Autodesk Fusion 360 part; units mm, degrees
sketch "Sketch1" plane through (0, 0, 0) normal (0, 0, 1) x (1, 0, 0)
  circle A0 centre (0, 0) radius 2.5
  dimension "d1" = 5
extrude "Extrude1" add sketch "Sketch1" along normal blind 20
sketch "Sketch2" plane through (0, 0, 20) normal (0, 0, 1) x (-1, 0, 0)
  circle A0 centre (0, 0) radius 2.5
  line L0 (-2.3094, 4) -> (-4.6188, 0)
  line L1 (-4.6188, 0) -> (-2.3094, -4)
  line L2 (-2.3094, -4) -> (2.3094, -4)
  line L3 (2.3094, -4) -> (4.6188, 0)
  line L4 (4.6188, 0) -> (2.3094, 4)
  line L5 (2.3094, 4) -> (-2.3094, 4)
  dimension "d4" = 4
extrude "Extrude2" add sketch "Sketch2" along normal blind 4 contours A0 | L0 L1 L2 L3 L4 L5
thread "Thread1"
Geometry: final body of the model. Coordinates: model frame, mm. A direction names the side the tool comes from. Round coordinates to 2 decimals unless told otherwise and drop trailing zeros. Loops run counter-clockwise (first coordinate to the right, second up) from the corner with the lowest first, then second, coordinate; pieces in that order, holes last. Notation, with made-up numbers: M 18.5,1.25 L 53.5,1.25 A12 ccw 53.5,24.25 Z; hole C 52.25,-27 d9. An arc over 180 degrees is marked long. One line per question, with ' | ' between items.
(1) Contact query for flat-ended pins moving along their axis: P1, Ø5, axis at x = 3, z = 11.5, coming from the +Y side; P2, Ø5, axis at x = -1.5, z = 13.5, coming from the -Y side; P3, Ø4, axis at x = -3, z = 8, coming from the +Y side. Output: stop coordinate, or through.
Check result:
P1: stops at y = 2.45 | P2: stops at y = -2.5 | P3: stops at y = 2.29
(2) Cut plane C-C on y = -1. Return the cut outline in (x, z), plus the area to 3 significant figures.
Check result:
outline: M -4.04,20 L -2.29,20 L -2.29,0 L 2.29,0 L 2.29,20 L 4.04,20 L 4.04,24 L -4.04,24 Z | area: 124 mm2
(3) Access query for faces 1 (the flat face through (-2, -2, 20)), 2 (the flat face through (0, 4, 22)). Directions: +Z, -Z, +X, -X, +Y, -Y. A direction counts if a zero-diameter tool reaches every point of the face in a straight line with its end or side. Return the directions, or none.
Check result:
face 1: -Z | face 2: +Z, -Z, +X, -X, +Y
(4) Material intervals for line 1 along Z through (x, y) = (2.25, 2.5); line 2 along Y through (x, z) = (1, 4.75); line 3 along X through (y, z) = (1.75, 9.5), sorted ascending. Write a range as from..to.
Check result:
line 1: z = 20..24 | line 2: y = -2.29..2.29 | line 3: x = -1.79..1.79
(5) Cut plane D-D on z = 3.25. Return the cut outline in (x, y).
Check result:
outline: C 0,0 d5
(6) Cut plane A-A on x = 0. Return the cut outline in (y, z), plus the area to 3 significant figures.
Check result:
outline: M -4,20 L -2.5,20 L -2.5,0 L 2.5,0 L 2.5,20 L 4,20 L 4,24 L -4,24 Z | area: 132 mm2
(7) Cut plane B-B on z = 22.25. Return the cut outline in (x, y), plus the area to 3 significant figures.
Check result:
outline: M -4.62,0 L -2.31,-4 L 2.31,-4 L 4.62,0 L 2.31,4 L -2.31,4 Z | area: 55.4 mm2
